Check sheet for the drawn part. Datum: minimum x, y, z corner. Units: mm. Give positions to 0.01 mm unless a question says otherwise; leave off trailing zeros. Answer as a JSON object with one key per item and string values. Group by question number.
Item 1: Sectioned sample at A-A, the plane z = 133.35. Count the separate pieces of the cut face and the enclosed holes in it.
Item 2: Go/stop test with a flat-tipped pin: pin 1 (4 mm diameter, centred on x = 139.7, z = 57.15, fed in from +Y). Record where the tip stops, or that it passes through.
Item 3: Scan lines: line 1 along Z through (x, y) = (139.7, 5.05); line 2 along X through (y, z) = (4.5, 133.35); line 3 along X through (y, z) = (1.5, 19) (1 decimal). Record each from-to range of solid material in increasing order. Write a range as [from, to].
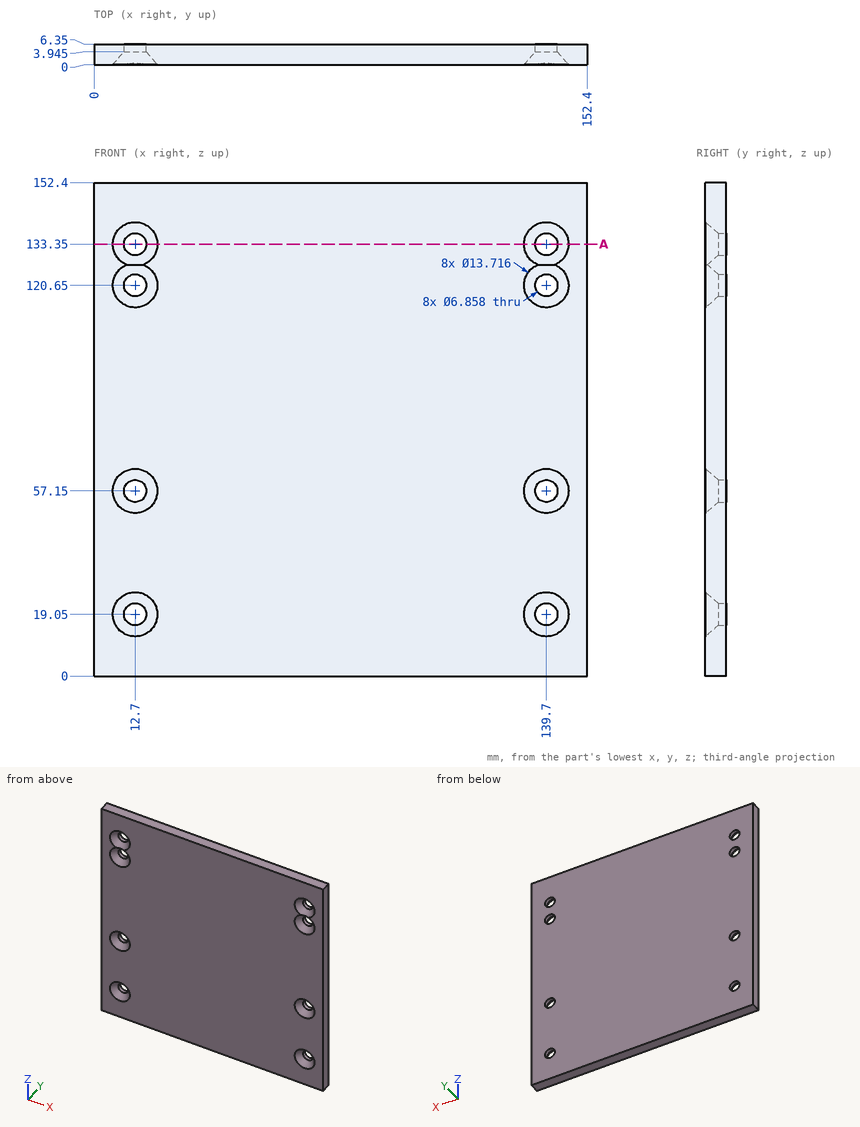
Geometry check:
{
 "1": {"separate pieces": "3", "enclosed holes": "0"},
 "2": {"pin 1": "through"},
 "3": {"line 1": "[0, 15.62], [22.48, 53.72], [60.58, 117.22], [124.08, 129.92], [136.78, 152.4]", "line 2": "[0, 9.27], [16.13, 136.27], [143.13, 152.4]", "line 3": "[0, 7.1], [18.3, 134.1], [145.3, 152.4]"}
}
